Could you check a few things on this model? Use its own coordinates, in mm. Face numbers are marked on the shaded views. A direction names the side the tool comes from. Round coordinates to 2 decimals unless told otherwise and drop trailing zeros. Answer as CSV lines item,"result". Start each with the question number.
Q1. Imagine slicing it at A-A on z = -3.25. Give the number of separate pieces and of enclosed holes in the cut face, and give its area (3 significant figures).
Q2. Will these pins go through, and if not, where does the flat tip stop? pin 1 Ø5 at (x, y) = (16, 16) entering from -Z; pin 2 Ø4 at (x, y) = (16, -16) entering from -Z; pin 3 Ø23 at (x, y) = (0, 0) entering from -Z.
Q3. For the marked faces 5, 6 and 7, which set-ups out of +Z, -Z, +X, -X, +Y, -Y let a thin tool reach every point of the face, with its end or its side?
Q4. If we mould it in two halves opening along Y, with no side actions, what happens to the marked faces 1, 2, 3 and 4? For each: pulls with the +Y half, pulls with the -Y half, needs draft (parallel to the pull), parting line crosses it, or undercut.
Q5. If I drill on line 1 (Y direction, x = -16, z = -2.25); line 2 (X direction, y = -14.5, z = -1.75); line 3 (X direction, y = 3.5, z = -0.25), over which ranges is the centre line in solid material (lowest first)? Write a range as [from, to].
from build123d import *

# Parameters (mm, degrees)
SKETCH1_R           = 19
SKETCH1_R_2         = 2.15
BOSS_EXTRUDE1_DEPTH = 5
BOSS_EXTRUDE2_DEPTH = 4


with BuildPart() as part:
    # Sketch1 → Boss-Extrude1 (new, symmetric)
    with BuildSketch(Plane.XY):
        with BuildLine():
            ThreePointArc((-20, 18), (-19.414213562, 19.414213562), (-18, 20))
            Line((-18, 20), (18, 20))
            ThreePointArc((18, 20), (19.414213562, 19.414213562), (20, 18))
            Line((20, 18), (20, -18))
            ThreePointArc((20, -18), (19.414213562, -19.414213562), (18, -20))
            Line((18, -20), (-18, -20))
            ThreePointArc((-18, -20), (-19.414213562, -19.414213562), (-20, -18))
            Line((-20, -18), (-20, 18))
        make_face()
        Circle(SKETCH1_R, mode=Mode.SUBTRACT)
        with Locations((-16, -16)):
            Circle(SKETCH1_R_2, mode=Mode.SUBTRACT)
        with Locations((16, -16)):
            Circle(SKETCH1_R_2, mode=Mode.SUBTRACT)
        with Locations((16, 16)):
            Circle(SKETCH1_R_2, mode=Mode.SUBTRACT)
        with Locations((-16, 16)):
            Circle(SKETCH1_R_2, mode=Mode.SUBTRACT)
    extrude(amount=BOSS_EXTRUDE1_DEPTH, both=True)

    # Sketch1_5 → Boss-Extrude2 (add, symmetric)
    with BuildSketch(Plane.XY):
        with BuildLine():
            add(Edge.make_bspline(
                [(2.949489743, 0.548188159), (8.845203175, 8.391149402), (17.92289399, 6.306335785)],
                knots=[0, 0, 0, 1, 1, 1], degree=2))
            ThreePointArc((17.92289399, 6.306335785), (16.454482672, 9.5), (14.42289399, 12.368513612))
            add(Edge.make_bspline(
                [(1.949489743, 2.280238966), (5.266917454, 11.646464502), (14.42289399, 12.368513612)],
                knots=[0, 0, 0, 1, 1, 1], degree=2))
            ThreePointArc((1.949489743, 2.280238966), (1.5, 2.598076211), (1, 2.828427125))
            add(Edge.make_bspline(
                [(1, 2.828427125), (-1.258927409, 8.1328538), (0, 12.674849397)],
                knots=[0, 0, 0, 0.587597174, 0.587597174, 0.587597174], degree=2))
            add(Edge.make_bspline(
                [(0, 12.674849397), (0.883573382, 15.862631615), (3.5, 18.674849397)],
                knots=[0.587597174, 0.587597174, 0.587597174, 1, 1, 1], degree=2))
            ThreePointArc((3.5, 18.674849397), (0, 19), (-3.5, 18.674849397))
            add(Edge.make_bspline(
                [(-1, 2.828427125), (-7.452675396, 10.384516566), (-3.5, 18.674849397)],
                knots=[0, 0, 0, 1, 1, 1], degree=2))
            ThreePointArc((-1, 2.828427125), (-1.5, 2.598076211), (-1.949489743, 2.280238966))
            add(Edge.make_bspline(
                [(-1.949489743, 2.280238966), (-11.689550136, 3.46459595), (-14.42289399, 12.368513612)],
                knots=[0, 0, 0, 1, 1, 1], degree=2))
            ThreePointArc((-14.42289399, 12.368513612), (-16.454482672, 9.5), (-17.92289399, 6.306335785))
            add(Edge.make_bspline(
                [(-2.949489743, 0.548188159), (-12.71959285, -1.261947936), (-17.92289399, 6.306335785)],
                knots=[0, 0, 0, 1, 1, 1], degree=2))
            ThreePointArc((-2.949489743, 0.548188159), (-3, 0), (-2.949489743, -0.548188159))
            add(Edge.make_bspline(
                [(-2.949489743, -0.548188159), (-8.845203175, -8.391149402), (-17.92289399, -6.306335785)],
                knots=[0, 0, 0, 1, 1, 1], degree=2))
            ThreePointArc((-17.92289399, -6.306335785), (-16.454482672, -9.5), (-14.42289399, -12.368513612))
            add(Edge.make_bspline(
                [(-1.949489743, -2.280238966), (-5.266917454, -11.646464502), (-14.42289399, -12.368513612)],
                knots=[0, 0, 0, 1, 1, 1], degree=2))
            ThreePointArc((-1.949489743, -2.280238966), (-1.5, -2.598076211), (-1, -2.828427125))
            add(Edge.make_bspline(
                [(-1, -2.828427125), (2.844346961, -11.855745352), (-3.5, -18.674849397)],
                knots=[0, 0, 0, 1, 1, 1], degree=2))
            ThreePointArc((-3.5, -18.674849397), (0, -19), (3.5, -18.674849397))
            add(Edge.make_bspline(
                [(1, -2.828427125), (7.452675396, -10.384516566), (3.5, -18.674849397)],
                knots=[0, 0, 0, 1, 1, 1], degree=2))
            ThreePointArc((1, -2.828427125), (1.5, -2.598076211), (1.949489743, -2.280238966))
            add(Edge.make_bspline(
                [(1.949489743, -2.280238966), (11.689550136, -3.46459595), (14.42289399, -12.368513612)],
                knots=[0, 0, 0, 1, 1, 1], degree=2))
            ThreePointArc((14.42289399, -12.368513612), (16.454482672, -9.5), (17.92289399, -6.306335785))
            add(Edge.make_bspline(
                [(2.949489743, -0.548188159), (12.71959285, 1.261947936), (17.92289399, -6.306335785)],
                knots=[0, 0, 0, 1, 1, 1], degree=2))
            ThreePointArc((2.949489743, -0.548188159), (3, 0), (2.949489743, 0.548188159))
        make_face()
    extrude(amount=BOSS_EXTRUDE2_DEPTH, both=True)


solid = part.part
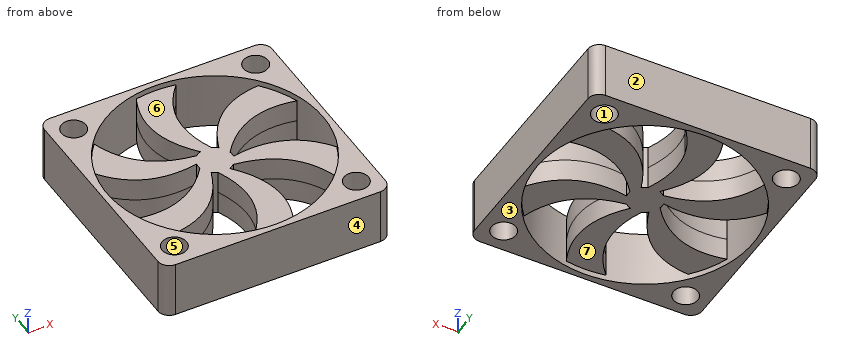
Checks:
1,separate pieces,"1"
1,enclosed holes,"10"
1,area,"868 mm^2"
2,pin 1,"z = -5"
2,pin 2,"through"
2,pin 3,"z = -4"
3,face 5,"+Z, -Z"
3,face 6,"+Z"
3,face 7,"-Z"
4,face 1,"undercut"
4,face 2,"pulls with the +Y half"
4,face 3,"needs draft"
4,face 4,"pulls with the -Y half"
5,line 1,"[-20, -18.15], [-13.85, -6.64], [3.98, 13.85], [18.15, 20]"
5,line 2,"[-20, -17.54], [-14.46, -12.28], [-0.66, 4.84], [12.28, 14.46], [17.54, 20]"
5,line 3,"[-20, -18.67], [-15.49, -6.74], [-1.55, 0.73], [2.42, 5.68], [18.67, 20]"
